Check sheet for the modelled part. Datum: model origin and axes. Units: mm. Coordinates: 2 decimals unless noted, no trailing zeros. Write each loop counter-clockwise with the first axis right and the second up, starting at its lowest first coordinate (ties: lowest second). Pieces come first, ordered by that corner, then holes. Notation, with made-up numbers: M -18.5,67.25 L 39.5,67.25 A34 cw 39.5,99.25 Z; hole C 35.25,52.25 d5. An arc over 180 degrees is marked long. Answer as CSV lines item,"result". Start each with the question number.
Q1. Sectioned sample at C-C, the plane y = 1.75. Count the separate pieces of the cut face and the enclosed holes in it, then the cut area to 3 significant figures.
Q2. Sectioned sample at A-A, the plane x = 85. Record the cut outline in (y, z).
Q3. Sectioned sample at B-B, the plane z = 73.5. Record the cut outline in (x, y).
Q4. Depth check by flat-ended pin: pin 1 Ø6 at (x, z) = (12, 73) entering from -Y. Enter the tip coordinate at first touch or a pass-through.
Q5. Thickness scan on line 1 along Z through (x, y) = (88, 1.15); line 2 along X through (y, z) = (1.9, 6); line 3 along Z through (x, y) = (-77, 0.2). Record the ranges inside material, lowest first. Write a range as from..to.
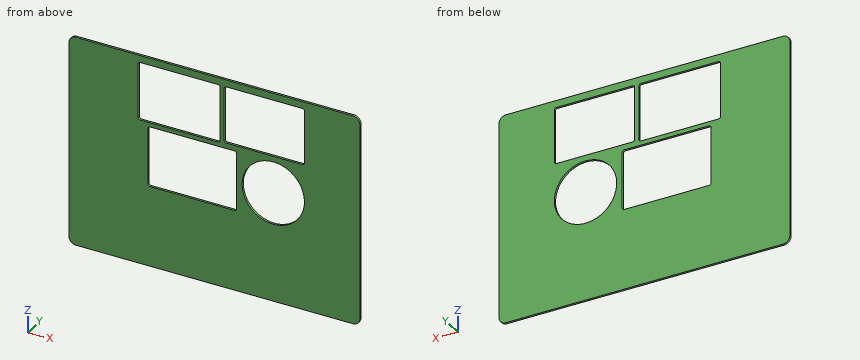
from build123d import *

# Parameters (mm, degrees)
SKETCH_2_W      = 420
SKETCH_2_H      = 300
SKETCH_2_R      = 45
SKETCH_2_W_2    = 116
SKETCH_2_H_2    = 81
SKETCH_2_W_3    = 118
SKETCH_2_H_3    = 83
SKETCH_2_W_4    = 128
SKETCH_2_H_4    = 86
EXTRUDE_2_DEPTH = 3
FILLET_1_R      = 3
FILLET_2_R      = 3
FILLET_3_R      = 3
FILLET_4_R      = 3
FILLET_5_R      = 3
FILLET_6_R      = 3
FILLET_7_R      = 3
FILLET_8_R      = 3
FILLET_9_R      = 3
FILLET_10_R     = 3
FILLET_11_R     = 3
FILLET_12_R     = 3
FILLET_13_R     = 10
FILLET_14_R     = 10
FILLET_15_R     = 10
FILLET_16_R     = 10


with BuildPart() as part:
    # 草图2 → 凸台-拉伸2 (new body)
    with BuildSketch(Plane(origin=(0, 0, 0), x_dir=(1, 0, 0), z_dir=(0, 1, 0))):
        Rectangle(SKETCH_2_W, SKETCH_2_H)
        with Locations(Location((85, -6, 0), (0, 0, 270))):
            Circle(SKETCH_2_R, mode=Mode.SUBTRACT)
        with Locations((72, -99.5)):
            Rectangle(SKETCH_2_W_2, SKETCH_2_H_2, mode=Mode.SUBTRACT)
        with Locations((-51, -98.5)):
            Rectangle(SKETCH_2_W_3, SKETCH_2_H_3, mode=Mode.SUBTRACT)
        with Locations((-32, -8)):
            Rectangle(SKETCH_2_W_4, SKETCH_2_H_4, mode=Mode.SUBTRACT)
    extrude(amount=EXTRUDE_2_DEPTH)

    # 圆角1
    fillet_1_edges = [part.edges().sort_by_distance(p)[0] for p in [
        (-96, 1.5, -35),
    ]]
    fillet(fillet_1_edges, radius=FILLET_1_R)

    # 圆角2
    fillet_2_edges = [part.edges().sort_by_distance(p)[0] for p in [
        (-96, 1.5, 51),
    ]]
    fillet(fillet_2_edges, radius=FILLET_2_R)

    # 圆角3
    fillet_3_edges = [part.edges().sort_by_distance(p)[0] for p in [
        (32, 1.5, 51),
    ]]
    fillet(fillet_3_edges, radius=FILLET_3_R)

    # 圆角4
    fillet_4_edges = [part.edges().sort_by_distance(p)[0] for p in [
        (32, 1.5, -35),
    ]]
    fillet(fillet_4_edges, radius=FILLET_4_R)

    # 圆角5
    fillet_5_edges = [part.edges().sort_by_distance(p)[0] for p in [
        (14, 1.5, 140),
    ]]
    fillet(fillet_5_edges, radius=FILLET_5_R)

    # 圆角6
    fillet_6_edges = [part.edges().sort_by_distance(p)[0] for p in [
        (14, 1.5, 59),
    ]]
    fillet(fillet_6_edges, radius=FILLET_6_R)

    # 圆角7
    fillet_7_edges = [part.edges().sort_by_distance(p)[0] for p in [
        (130, 1.5, 59),
    ]]
    fillet(fillet_7_edges, radius=FILLET_7_R)

    # 圆角8
    fillet_8_edges = [part.edges().sort_by_distance(p)[0] for p in [
        (130, 1.5, 140),
    ]]
    fillet(fillet_8_edges, radius=FILLET_8_R)

    # 圆角9
    fillet_9_edges = [part.edges().sort_by_distance(p)[0] for p in [
        (8, 1.5, 140),
    ]]
    fillet(fillet_9_edges, radius=FILLET_9_R)

    # 圆角10
    fillet_10_edges = [part.edges().sort_by_distance(p)[0] for p in [
        (8, 1.5, 57),
    ]]
    fillet(fillet_10_edges, radius=FILLET_10_R)

    # 圆角11
    fillet_11_edges = [part.edges().sort_by_distance(p)[0] for p in [
        (-110, 1.5, 140),
    ]]
    fillet(fillet_11_edges, radius=FILLET_11_R)

    # 圆角12
    fillet_12_edges = [part.edges().sort_by_distance(p)[0] for p in [
        (-110, 1.5, 57),
    ]]
    fillet(fillet_12_edges, radius=FILLET_12_R)

    # 圆角13
    fillet_13_edges = [part.edges().sort_by_distance(p)[0] for p in [
        (-210, 1.5, 150),
    ]]
    fillet(fillet_13_edges, radius=FILLET_13_R)

    # 圆角14
    fillet_14_edges = [part.edges().sort_by_distance(p)[0] for p in [
        (210, 1.5, 150),
    ]]
    fillet(fillet_14_edges, radius=FILLET_14_R)

    # 圆角15
    fillet_15_edges = [part.edges().sort_by_distance(p)[0] for p in [
        (210, 1.5, -150),
    ]]
    fillet(fillet_15_edges, radius=FILLET_15_R)

    # 圆角16
    fillet_16_edges = [part.edges().sort_by_distance(p)[0] for p in [
        (-210, 1.5, -150),
    ]]
    fillet(fillet_16_edges, radius=FILLET_16_R)


solid = part.part
Output:
1,separate pieces,"1"
1,enclosed holes,"4"
1,area,"89,400 mm^2"
2,outline,"M 0,-150 L 3,-150 L 3,-39 L 0,-39 Z; M 0,51 L 3,51 L 3,59 L 0,59 Z; M 0,140 L 3,140 L 3,150 L 0,150 Z"
3,outline,"M -210,0 L -110,0 L -110,3 L -210,3 Z; M 8,0 L 14,0 L 14,3 L 8,3 Z; M 130,0 L 210,0 L 210,3 L 130,3 Z"
4,pin 1,"stops at y = 0"
5,line 1,"z = -150..-38.9, 50.9..59, 140..150"
5,line 2,"x = -210..-96, 32..40, 130..210"
5,line 3,"z = -150..-35, 51..57, 140..150"
